Build history of the part. All positions in model axes, mm. A direction names the side the tool comes from. Give positions to 0.01 mm unless a question says otherwise; leave off trailing zeros. Loops run counter-clockwise (first coordinate to the right, second up) from the corner with the lowest first, then second, coordinate; pieces in that order, holes last. Notation, with made-up numbers: M 52.25,-8.5 L 84.25,-8.5 A25 ccw 84.25,14.5 Z; hole C -9.5,63 d7. An arc over 180 degrees is marked long. Answer as a JSON object with one key per item and string values. Group by question number.
1. Drill centre lines: line 1 along Z through (x, y) = (28, -30.5); line 2 along Y through (x, z) = (141, 3.5); line 3 along X through (y, z) = (-0.5, 3.25). Where is each one in solid material? Low to high. Write a range as [from, to].
2. Drop flat-ended pins along their axis: pin 1 Ø10 at (x, y) = (147, 0.5) entering from +Z; pin 2 Ø5.5 at (x, z) = (129, 6.5) entering from +Y; pin 3 Ø8 at (x, y) = (51.5, 10) entering from +Z; pin 4 Ø2 at (x, z) = (86.5, 3.5) entering from -Y. Give the stop position or say it passes through.
3. Slice it at B-B (x = 162). List the corners of the cut face in (y, z), then the cut area to 3 significant figures.
4. Slice it at C-C (y = -31). List the corners of the cut face in (x, z), then the cut area to 3 significant figures.
5. 3-axis set-ups, long thin cutter, end or side, ignore diameter. For faces 1 (the face through (136, -29, 5)), 2 (the face through (136, 11, 5)), 3 (the face through (91, -4, 0)): which of +Z, -Z, +X, -X, +Y, -Y reach the whole face in a straight line?
6. Slice it at A-A (y = -6). List the corners of the cut face in (x, z).
from build123d import *

# Parameters (mm, degrees)
BOSS_EXTRUDE1_DEPTH = 3
SKETCH2_W           = 120
SKETCH2_H           = 40
BOSS_EXTRUDE2_DEPTH = 12
CUT_EXTRUDE1_REACH  = 189.417
FILLET1_R           = 10
FILLET2_R           = 4


with BuildPart() as part:
    # Sketch1 → Boss-Extrude1 (new body)
    with BuildSketch(Plane.XY):
        with BuildLine():
            Line((180, 0), (180, -39))
            Line((180, -39), (0, -39))
            Line((0, -39), (0, 0))
            ThreePointArc((0, 0), (90, 50), (180, 0))
        make_face()
    extrude(amount=BOSS_EXTRUDE1_DEPTH)

    # Sketch2 → Boss-Extrude2 (add)
    with BuildSketch(Plane.XY.offset(3)):
        with Locations((90, -9)):
            Rectangle(SKETCH2_W, SKETCH2_H)
    extrude(amount=BOSS_EXTRUDE2_DEPTH)

    # Sketch3 → Cut-Extrude1 (cut, up to next)
    with BuildSketch(Plane(origin=(0, 11, 0), x_dir=(1, 0, 0), z_dir=(0, 1, 0)), mode=Mode.PRIVATE) as cut_extrude1_sk1:
        with BuildLine():
            Line((30, -15), (150, -15))
            ThreePointArc((150, -15), (90, -5.870751133), (30, -15))
        make_face()
    cut_extrude1_tool1 = extrude(cut_extrude1_sk1.sketch, amount=-CUT_EXTRUDE1_REACH, mode=Mode.PRIVATE) & part.part
    add(cut_extrude1_tool1.solids().sort_by_distance((90, 11, 11.341124))[0], mode=Mode.SUBTRACT)

    # Fillet1
    # the kernel refuses this fillet: 10 mm, written as the material it takes off along each edge
    with BuildSketch(Plane(origin=(150, 42.911423728, 15), x_dir=(0, 0, -1), z_dir=(0, -1, 0)), Plane(origin=(30, -60.911423728, 15), x_dir=(0, 0, -1), z_dir=(0, 1, 0))) as fillet1_piece_1:
        with BuildLine():
            CenterArc((13.125456564, -9.936465545), FILLET1_R, 96.462082414, 97.214818073)
            Line((3.409011311, -12.300929891), (3.214682406, -12.348219178))
            ThreePointArc((3.214682406, -12.348219178), (1.609086457, -6.176908891), (-0.190949181, -0.059484539))
            Line((-0.190949181, -0.059484539), (0, 0.2))
            ThreePointArc((0, 0.2), (6, 0.2), (11.977490869, 0.198729311))
            Line((11.977490869, 0.198729311), (12, 0))
        make_face()
    extrude(amount=103.822847456, mode=Mode.SUBTRACT)

    # Fillet2
    fillet2_edges = [part.edges().sort_by_distance(p)[0] for p in [
        (90, -29, 5.870751133),
        (90, 11, 5.870751133),
        (34.210640521, 11, 10.073014501),
        (145.789359479, 11, 10.073014501),
        (34.210640521, -29, 10.073014501),
        (145.789359479, -29, 10.073014501),
    ]]
    fillet(fillet2_edges, radius=FILLET2_R)


solid = part.part
Established:
{
 "1": {"line 1": "z = [0, 3]", "line 2": "y = [-29, 11]", "line 3": "x = [30.03, 149.97]"},
 "2": {"pin 1": "stops at z = 11.69", "pin 2": "stops at y = 11", "pin 3": "stops at z = 10.18", "pin 4": "stops at y = -39"},
 "3": {"outline": "M -39,0 L 21.79,0 L 21.79,3 L -39,3 Z", "area": "182 mm^2"},
 "4": {"outline": "M 0,0 L 180,0 L 180,3 L 0,3 Z", "area": "540 mm^2"},
 "5": {"face 1": "+Z, +X, -X, -Y", "face 2": "+Z, +X, -X, +Y", "face 3": "-Z, +X, -X, +Y, -Y"},
 "6": {"outline": "M 0,0 L 180,0 L 180,3 L 150,3 A10 ccw 137.7,11.59 A201.73 cw 42.3,11.59 A10 ccw 30,3 L 0,3 Z"}
}
